```python
from build123d import *

# Parameters (mm, degrees)
EXTRUDE_1_DEPTH     = 50
SKETCH_2_R          = 5
CUT_EXTRUDE_1_DEPTH = 55.772255751
SKETCH_3_W          = 40
SKETCH_3_H          = 10
EXTRUDE_3_DEPTH     = 15
CUT_EXTRUDE_2_DEPTH = 48.16990566


with BuildPart() as part:
    # 草图1 → 凸台-拉伸1 (new body)
    with BuildSketch(Plane.XY):
        Polygon((-20, 0), (20, 0), (20, -5), (10.5, -5), (14, -10), (-14, -10), (-10.5, -5), (-20, -5), align=None)
    extrude(amount=EXTRUDE_1_DEPTH)

    # 草图2 → 切除-拉伸1 (cut, through all)
    with BuildSketch(Plane(origin=(0, 0, 0), x_dir=(1, 0, 0), z_dir=(0, 1, 0))):
        with Locations(Location((0, -32, 0), (0, 0, 270))):
            Circle(SKETCH_2_R)
    extrude(amount=-CUT_EXTRUDE_1_DEPTH, mode=Mode.SUBTRACT)

    # 草图3 → 凸台-拉伸3 (add)
    with BuildSketch(Plane(origin=(0, 0, 0), x_dir=(1, 0, 0), z_dir=(0, 1, 0))):
        with Locations((0, -5)):
            Rectangle(SKETCH_3_W, SKETCH_3_H)
    extrude(amount=EXTRUDE_3_DEPTH)

    # 草图4 → 切除-拉伸2 (cut, through all)
    with BuildSketch(Plane.XY.offset(10)):
        with BuildLine():
            Line((-12, 15), (12, 15))
            ThreePointArc((12, 15), (0, 3), (-12, 15))
        make_face()
    extrude(amount=-CUT_EXTRUDE_2_DEPTH, mode=Mode.SUBTRACT)


solid = part.part
```
Input: part model. Units: mm. Frame: model coordinates. A direction names the side the tool comes from. Give positions to 0.01 mm unless a question says otherwise; leave off trailing zeros. Loops run counter-clockwise (first coordinate to the right, second up) from the corner with the lowest first, then second, coordinate; pieces in that order, holes last.
1) Line query: L1, parallel to X at y = -3.75, z = 32; L2, parallel to Y at x = -9.5, z = 17; L3, parallel to Y at x = 15.5, z = 36. Output: solid intervals per line, ascending.
A:
L1: x = -20 to -5, 5 to 20
L2: y = -10 to 0
L3: y = -5 to 0
2) Section query C-C on y = 9.5. Return the cut outline in (x, z), and give its area (3 significant figures).
A:
outline: (-20, 0) - (-10.67, 0) - (-10.67, 10) - (-20, 10) - close; (10.67, 0) - (20, 0) - (20, 10) - (10.67, 10) - close
area: 187 mm2
3) Mould query, pull axis X, two halves, no side actions, for faces 4 (the flat face through (-16, 15, 5)), 5 (the cylindrical face through (0, 3, 5)), 6 (the flat face through (-20, -2, 14)), 7 (the cylindrical face through (0, -5, 27)). Classes: released by +X, released by -X, zero draft, split by the parting line, or undercut.
A:
face 4: zero draft
face 5: undercut
face 6: released by -X
face 7: undercut
4) Section query A-A on x = 0. Return the cut outline in (y, z), and give its area (3 significant figures).
A:
outline: (-10, 0) - (3, 0) - (3, 10) - (0, 10) - (0, 27) - (-10, 27) - close; (-10, 37) - (0, 37) - (0, 50) - (-10, 50) - close
area: 430 mm2
5) Section query D-D on z = 25.5. Return the cut outline in (x, y).
A:
outline: (-20, -5) - (-10.5, -5) - (-14, -10) - (14, -10) - (10.5, -5) - (20, -5) - (20, 0) - (-20, 0) - close
6) Reachability of faces 1 (the flat face through (15, -5, 25)), 2 (the flat face through (-5, 0, 30)), 3 (the flat face through (-15, -5, 25)) from +Z, -Z, +X, -X, +Y, -Y: full face, straight path, thin tool, end or side. Return the list, or none.
A:
face 1: +Z, -Z, +X
face 2: +Z, +X, -X, +Y
face 3: +Z, -Z, -X
7) Contact query for flat-ended pins moving along their axis: pin 1 (13 mm diameter, centred on x = 0, z = 32, fed in from +Y); pin 2 (6 mm diameter, centred on x = 7.5, z = 9, fed in from +Y); pin 3 (1 mm diameter, centred on y = -7.5, z = 19.5, fed in from -X). Output: stop coordinate, or through.
A:
pin 1: stops at y = 0
pin 2: stops at y = 9.19
pin 3: stops at x = -12.6
8) Section query B-B on z = 32. Return the cut outline in (x, y), and give its area (4 significant figures).
A:
outline: (-20, -5) - (-10.5, -5) - (-14, -10) - (-5, -10) - (-5, 0) - (-20, 0) - close; (5, -10) - (14, -10) - (10.5, -5) - (20, -5) - (20, 0) - (5, 0) - close
area: 222.5 mm2
